Verification items for the finished model (mm, model axes). Face numbers are marked on the shaded views. A direction names the side the tool comes from. Coordinates: 2 decimals unless noted, no trailing zeros. Order: outer loops, then holes, each group sorted by start corner. A loop starts at its lowest first (then second) coordinate and runs counter-clockwise, first axis right, second up. Notation, with made-up numbers: M 5.25,-37 L 59.25,-37 A14 ccw 59.25,-18 Z; hole C 15,87 d9. An arc over 180 degrees is marked long. Return JSON: item names as keys, results as strings. Group by question number.
Q1. Section check A-A, the plane x = 0. Enter the section's corners in (y, z).
Q2. Go/stop test with flat-tipped pins: pin 1 Ø3 at (y, z) = (12, 3) entering from +X; pin 2 Ø1.2 at (y, z) = (12.5, 4) entering from -X; pin 3 Ø1.5 at (x, y) = (-9, 1) entering from +Z. Record where each tip stops, or that it passes through.
Q3. Section check D-D, the plane x = 6.5. Enter the section's corners in (y, z), then the cut area to 3 significant figures.
Q4. Section check B-B, the plane y = 0. Enter the section's corners in (x, z).
Q5. Access from +Z, -Z, +X, -X, +Y, -Y to the whole of each face (thin tool, end or side, straight path). Record for the marked faces 1 and 2.
Q6. Thickness scan on probe 1 along Y at (x, z) = (0, 0.65); probe 2 along Z at (x, y) = (5, 3.5); probe 3 along Y at (x, z) = (-2, 3.4). Record the ranges inside material, lowest first.
Q7. Section check C-C, the plane z = 0.5. Enter the section's corners in (x, y), then the cut area to 3 significant figures.
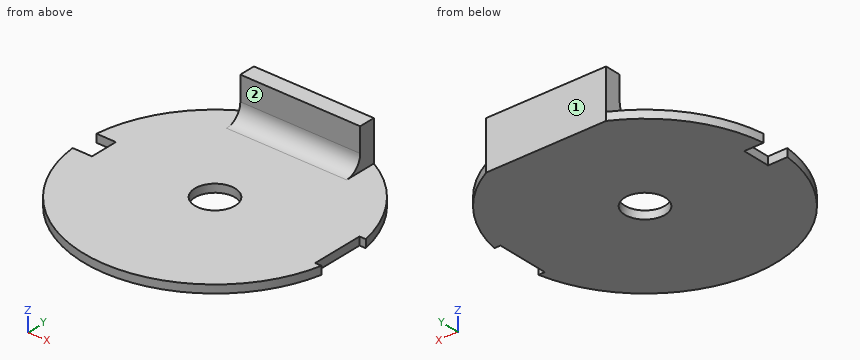
from build123d import *

# Parameters (mm, degrees)
SKETCH_1_R          = 2.5
EXTRUDE_1_DEPTH     = 1
SKETCH_2_W          = 5
SKETCH_2_H          = 3.5
SKETCH_2_W_2        = 2
SKETCH_2_H_2        = 6.5
CUT_EXTRUDE_1_DEPTH = 2
SKETCH_3_W          = 14.891608376
SKETCH_3_H          = 2
EXTRUDE_2_DEPTH     = 5
FILLET_1_R          = 2


with BuildPart() as part:
    # 草图1 → 凸台-拉伸1 (new body)
    with BuildSketch(Plane.XY):
        with BuildLine():
            Line((-7.445804188, 14.5), (7.445804188, 14.5))
            ThreePointArc((7.445804188, 14.5), (0, -16.3), (-7.445804188, 14.5))
        make_face()
        Circle(SKETCH_1_R, mode=Mode.SUBTRACT)
    extrude(amount=EXTRUDE_1_DEPTH)

    # 草图2 → 切除-拉伸1 (cut, through all)
    with BuildSketch(Plane.XY.offset(1)):
        with Locations((-16.3, 0)):
            Rectangle(SKETCH_2_W, SKETCH_2_H)
        with Locations((16.2, 0)):
            Rectangle(SKETCH_2_W_2, SKETCH_2_H_2)
    extrude(amount=-CUT_EXTRUDE_1_DEPTH, mode=Mode.SUBTRACT)

    # 草图3 → 凸台-拉伸2 (add)
    with BuildSketch(Plane.XY.offset(1)):
        with Locations((0, 13.5)):
            Rectangle(SKETCH_3_W, SKETCH_3_H)
    extrude(amount=EXTRUDE_2_DEPTH)

    # 圆角1
    fillet_1_edges = [part.edges().sort_by_distance(p)[0] for p in [
        (0, 12.5, 1),
    ]]
    fillet(fillet_1_edges, radius=FILLET_1_R)


solid = part.part
Numbers:
{
 "1": {"outline": "M -16.3,0 L -2.5,0 L -2.5,1 L -16.3,1 Z; M 2.5,0 L 14.5,0 L 14.5,6 L 12.5,6 L 12.5,3 A2 cw 10.5,1 L 2.5,1 Z"},
 "2": {"pin 1": "stops at x = 7.45", "pin 2": "stops at x = -7.45", "pin 3": "stops at z = 1"},
 "3": {"outline": "M -14.95,0 L 14.5,0 L 14.5,6 L 12.5,6 L 12.5,3 A2 cw 10.5,1 L -14.95,1 Z", "area": "40.3 mm2"},
 "4": {"outline": "M -13.8,0 L -2.5,0 L -2.5,1 L -13.8,1 Z; M 2.5,0 L 15.2,0 L 15.2,1 L 2.5,1 Z"},
 "5": {"face 1": "+Z, -Z, +X, -X, +Y", "face 2": "+Z, +X, -X, -Y"},
 "6": {"probe 1": "y = -16.3 to -2.5, 2.5 to 14.5", "probe 2": "z = 0 to 1", "probe 3": "y = 12.5 to 14.5"},
 "7": {"outline": "M -16.21,-1.75 A16.3 ccw 15.97,-3.25 L 15.2,-3.25 L 15.2,3.25 L 15.97,3.25 A16.3 ccw 7.45,14.5 L -7.45,14.5 A16.3 ccw -16.21,1.75 L -13.8,1.75 L -13.8,-1.75 Z; hole C 0,0 d5", "area": "782 mm2"}
}
